from build123d import *

# Parameters (mm, degrees)
F1_DEPTH  = 17.3482
F3_DEPTH  = 17.3215080757
F5_DEPTH  = 17.3215080757
F7_DEPTH  = 17.3215080757
F8_T      = -1
F10_DEPTH = 1
F12_DEPTH = 1
F14_DEPTH = 1
F16_DEPTH = 1
F18_DEPTH = 1
F20_DEPTH = 1


with BuildPart() as f1:
    # F0 (on Top) → F1 (new body)
    with BuildSketch(Plane.XY):
        Polygon((0, 11.5470053838), (-10, -5.7735026919), (10, -5.7735026919), align=None)
    extrude(amount=F1_DEPTH)

    # F2 (on face) → F3 (cut, through all)
    with BuildSketch(Plane(origin=(-5, 2.8867513459, 0), x_dir=(-0.5, -0.8660254038, 0), z_dir=(-0.8660254038, 0.5, 0))):
        Polygon((-10, 17.3482), (-10, 0), (0, 17.3482), align=None)
        Polygon((10, 17.3482), (0, 17.3482), (10, 0), align=None)
    extrude(amount=-F3_DEPTH, mode=Mode.SUBTRACT)

    # F4 (on face) → F5 (cut, through all)
    with BuildSketch(Plane.XZ.offset(5.7735026919)):
        Polygon((-10, 17.3482), (-10, 0), (0, 17.3482), align=None)
        Polygon((10, 17.3482), (0, 17.3482), (10, 0), align=None)
    extrude(amount=-F5_DEPTH, mode=Mode.SUBTRACT)

    # F6 (on face) → F7 (cut, through all)
    with BuildSketch(Plane(origin=(5, 2.8867513459, 0), x_dir=(-0.5, 0.8660254038, 0), z_dir=(0.8660254038, 0.5, 0))):
        Polygon((-10, 17.3482), (-10, 0), (0, 17.3482), align=None)
        Polygon((10, 17.3482), (0, 17.3482), (10, 0), align=None)
    extrude(amount=-F7_DEPTH, mode=Mode.SUBTRACT)

    # F8
    f8_openings = [f1.faces().sort_by_distance(p)[0] for p in [
        (0, 0, 0),
    ]]
    offset(amount=F8_T, openings=f8_openings)

    # F9 (on face) → F10 (cut, through all)
    with BuildSketch(Plane(origin=(7.5059859034, 0, 4.326665535), x_dir=(0, 1, 0), z_dir=(0.8663709312, 0, 0.4994010509))):
        Polygon((-2.4401965598, 1.1524346291), (1.2200982799, 5.3840480932), (0, 9.6156615572), align=None)
    extrude(amount=-F10_DEPTH, mode=Mode.SUBTRACT)

    # F11 (on face) → F12 (cut, through all)
    with BuildSketch(Plane(origin=(3.7529929517, -6.5003744728, 4.326665535), x_dir=(0.9013048055, 0.3606091099, -0.240022327), z_dir=(0.4331854656, -0.7502992355, 0.4994010509))):
        Polygon((-2.6639553332, 9.2392796887), (-2.6639553332, 4.835282377), (2.0254065744, 1.7833656477), align=None)
    extrude(amount=-F12_DEPTH, mode=Mode.SUBTRACT)

    # F13 (on face) → F14 (cut, through all)
    with BuildSketch(Plane(origin=(-3.7529929517, -6.5003744728, 4.326665535), x_dir=(0.9013048055, -0.3606091099, 0.240022327), z_dir=(-0.4331854656, -0.7502992355, 0.4994010509))):
        Polygon((2.6639553332, 9.2392796887), (-2.0254065744, 1.7833656477), (2.6639553332, 4.835282377), align=None)
    extrude(amount=-F14_DEPTH, mode=Mode.SUBTRACT)

    # F15 (on face) → F16 (cut, through all)
    with BuildSketch(Plane(origin=(-7.5059859034, 0, 4.326665535), x_dir=(0, -1, 0), z_dir=(-0.8663709312, 0, 0.4994010509))):
        Polygon((-1.2200982799, 5.3840480932), (2.4401965598, 1.1524346291), (0, 9.6156615572), align=None)
    extrude(amount=-F16_DEPTH, mode=Mode.SUBTRACT)

    # F17 (on face) → F18 (cut, through all)
    with BuildSketch(Plane(origin=(3.7529929517, 6.5003744728, 4.326665535), x_dir=(-0.9013048055, 0.3606091099, 0.240022327), z_dir=(0.4331854656, 0.7502992355, 0.4994010509))):
        Polygon((2.6639553332, 9.2392796887), (0.3192743794, 5.5113226682), (2.6639553332, 0.4312850652), align=None)
    extrude(amount=-F18_DEPTH, mode=Mode.SUBTRACT)

    # F19 (on face) → F20 (cut, through all)
    with BuildSketch(Plane(origin=(-3.7529929517, 6.5003744728, 4.326665535), x_dir=(-0.9013048055, -0.3606091099, -0.240022327), z_dir=(-0.4331854656, 0.7502992355, 0.4994010509))):
        Polygon((-2.6639553332, 9.2392796887), (-2.6639553332, 0.4312850652), (-0.3192743794, 5.5113226682), align=None)
    extrude(amount=-F20_DEPTH, mode=Mode.SUBTRACT)


solid = f1.part
Build history of the part. All positions in model axes, mm. A direction names the side the tool comes from. Round coordinates to 2 decimals unless told otherwise and drop trailing zeros. Write each loop counter-clockwise with the first axis right and the second up, starting at its lowest first coordinate (ties: lowest second). Pieces come first, ordered by that corner, then holes. Notation, with made-up numbers: (-2.5, 6) -> (36.5, 6) arc R20 cw to (36.5, 45) -> close; hole circle Ø9 at (-4, 77.5). An arc over 180 degrees is marked (long way). Use one line per item in the form item = value.
Q1. Two-plate mould, pull along X, no slides. Class faces 1 (the flat face through (-4.5, 2.3, 0)), 2 (the flat face through (-4.93, 3.01, 3.31)), 3 (the flat face through (5.461, -0.636, 6.886)): released by +X, released by -X, zero draft, split by the parting line, or undercut.
Conclusion:
face_1 = zero draft
face_2 = released by -X
face_3 = undercut
Q2. Tool access for faces 4 (the flat face through (0, -4.774, 3)), 5 (the flat face through (1.138, -3.175, 10.604)), 6 (the flat face through (1.152, 5.563, 7.991)): list every direction of +Z, -Z, +X, -X, +Y, -Y with a clear straight run to the whole face (end or side of a thin tool).
Conclusion:
face_4 = -Z
face_5 = none
face_6 = +Z, +X, +Y
Q3. Band-saw the part on D-D, the plane y = 6.75. Write the cut outline in (x, z), then the cut area to 3 significant figures.
Conclusion:
outline = (-2.77, 0) -> (-1.61, 0) -> (-1.61, 3.8) -> (0, 5.2) -> (1.61, 3.8) -> (1.61, 0) -> (2.77, 0) -> (2.77, 4.8) -> (1.62, 5.8) -> (1.08, 5.01) -> (1.35, 6.03) -> (0, 7.21) -> (-1.35, 6.03) -> (-1.08, 5.01) -> (-1.62, 5.8) -> (-2.77, 4.8) -> close
area = 18.4 mm²
Q4. Band-saw the part on C-C, the plane x = -7.5. Write the cut outline in (y, z), then the cut area to 3 significant figures.
Conclusion:
outline = (-5.77, 0) -> (-4.77, 0) -> (-4.77, 1.67) -> (-4.33, 2.33) -> (-3.44, 2.33) -> (-3.44, 0) -> (-1.44, 0) -> (-1.44, 4.34) -> (-4.33, 4.34) -> (-5.77, 2.17) -> close
area = 14.3 mm²
Q5. Band-saw the part on B-B, the plane z = 14.75. Write the cut outline in (x, y), then the cut area to 3 significant figures.
Conclusion:
outline = (-1.5, -0.86) -> (0, -1.73) -> (1.5, -0.86) -> (1.5, 0.86) -> (0, 1.73) -> (-1.5, 0.86) -> close; hole (-0.34, -0.2) -> (0, -0.4) -> (0.34, -0.2) -> (0.34, 0.2) -> (0, 0.4) -> (-0.34, 0.2) -> close
area = 7.36 mm²
Q6. Drop flat-ended pins along their axis: P1, Ø4, axis at x = -2, z = 2.5, coming from the +Y side; P2, Ø3, axis at x = 6, z = 8, coming from the -Y side; P3, Ø2, axis at y = 5, z = 2.5, coming from the -X side. Give the stop position or say it passes through.
Conclusion:
P1 = 10.49
P2 = -4.08
P3 = -4.36
Q7. Band-saw the part on A-A, the plane y = 4. Write the cut outline in (x, z), then the cut area to 3 significant figures.
Conclusion:
outline = (-4.36, 0) -> (-3.2, 0) -> (-3.2, 6.56) -> (-2.35, 7.3) -> (-3.21, 8.55) -> (-4.36, 7.56) -> close; (-1.35, 10.17) -> (-0.92, 8.54) -> (0, 9.34) -> (0.92, 8.54) -> (1.35, 10.17) -> (0, 11.34) -> close; (2.35, 7.3) -> (3.2, 6.56) -> (3.2, 0) -> (4.36, 0) -> (4.36, 7.56) -> (3.21, 8.55) -> close
area = 24.9 mm²
Q8. Drill centre lines: L1, parallel to Y at x = -0.5, z = 10; L2, parallel to X at y = 0, z = 6.5; L3, parallel to Y at x = -1, z = 10.5. Where is each one in solid material? Low to high.
Conclusion:
L1 = -4.6 to -3.27, 3.27 to 4.6
L2 = -6.25 to -5.1, 5.1 to 6.25
L3 = -3.98 to -2.9, 2.9 to 3.98
